Design review of the part built by this model. Coordinates are the model's own, in mm. A direction names the side the tool comes from. Give positions to 0.01 mm unless a question says otherwise; leave off trailing zeros.
```python
from build123d import *

# Parameters (mm, degrees)
SKETCH1_W                        = 112
SKETCH1_H                        = 39
BOSS_EXTRUDE1_DEPTH              = 6
CUT_EXTRUDE1_REACH               = 70.505
TAP_DRILL_FOR_M3_TAP1_AT_2_COUNT = 2
TAP_DRILL_FOR_M3_TAP1_AT_2_PITCH = 30
FILLET1_R                        = 3
FILLET1_OF_MIRROR1_R             = 3
TAP_DRILL_FOR_M2_TAP1_D          = 1.6


with BuildPart() as part:
    # Sketch1 → Boss-Extrude1 (new body)
    with BuildSketch(Plane.XY):
        with Locations((0, 19.5)):
            Rectangle(SKETCH1_W, SKETCH1_H)
    extrude(amount=BOSS_EXTRUDE1_DEPTH)

    # Sketch2 → Cut-Extrude1 (cut, up to next)
    with BuildSketch(Plane.XY.offset(6), mode=Mode.PRIVATE) as cut_extrude1_sk1:
        Polygon((-56, 33), (-43.052558883, 33), (-29.196152423, 9), (-56, 9), align=None)
    cut_extrude1_tool1 = extrude(cut_extrude1_sk1.sketch, amount=-CUT_EXTRUDE1_REACH, mode=Mode.PRIVATE) & part.part
    # Sketch2 → Cut-Extrude1 (cut, up to next)
    with BuildSketch(Plane.XY.offset(6), mode=Mode.PRIVATE) as cut_extrude1_sk2:
        Polygon((-39.588457268, 39), (-37.856406461, 36), (-19.814954576, 36), (-10, 19), (0, 19), (0, 39), align=None)
    cut_extrude1_tool2 = extrude(cut_extrude1_sk2.sketch, amount=-CUT_EXTRUDE1_REACH, mode=Mode.PRIVATE) & part.part
    # Sketch2 → Cut-Extrude1 (cut, up to next)
    with BuildSketch(Plane.XY.offset(6), mode=Mode.PRIVATE) as cut_extrude1_sk3:
        Polygon((-56, 3), (-25.732050808, 3), (-24, 0), (-56, 0), align=None)
    cut_extrude1_tool3 = extrude(cut_extrude1_sk3.sketch, amount=-CUT_EXTRUDE1_REACH, mode=Mode.PRIVATE) & part.part
    # Sketch2 → Cut-Extrude1 (cut, up to next)
    with BuildSketch(Plane.XY.offset(6), mode=Mode.PRIVATE) as cut_extrude1_sk4:
        Polygon((-13.464101615, 13), (0, 13), (0, 6), (-20.535898385, 6), (-34.392304845, 30), (-23.279056191, 30), align=None)
    cut_extrude1_tool4 = extrude(cut_extrude1_sk4.sketch, amount=-CUT_EXTRUDE1_REACH, mode=Mode.PRIVATE) & part.part
    cut_extrude1_1 = cut_extrude1_tool1.solids().sort_by_distance((-45.659675, 19.60569, 6))[0]
    add(cut_extrude1_1, mode=Mode.SUBTRACT)
    cut_extrude1_2 = cut_extrude1_tool2.solids().sort_by_distance((-11.382019, 31.286174, 6))[0]
    add(cut_extrude1_2, mode=Mode.SUBTRACT)
    cut_extrude1_3 = cut_extrude1_tool3.solids().sort_by_distance((-40.428998, 1.486092, 6))[0]
    add(cut_extrude1_3, mode=Mode.SUBTRACT)
    cut_extrude1_4 = cut_extrude1_tool4.solids().sort_by_distance((-18.182863, 16.08438, 6))[0]
    add(cut_extrude1_4, mode=Mode.SUBTRACT)
    cut_extrude1 = cut_extrude1_1 + cut_extrude1_2 + cut_extrude1_3 + cut_extrude1_4  # Cut-Extrude1 as one shape, for the pattern or mirror that repeats it

    # Sketch3 → Tap Drill for M3 Tap1 (revolve, cut)
    with BuildSketch(Plane(origin=(-56, 36, 3), x_dir=(0, 0, 1), z_dir=(0, 1, 0))):
        Polygon((0, 0), (0, 10.751075774), (1.25, 10), (1.25, 0), align=None)
    tap_drill_for_m3_tap1 = revolve(axis=Axis((-62.35, 36, 3), (1, 0, 0)), mode=Mode.SUBTRACT)

    # Tap Drill for M3 Tap1 at 2: Tap Drill for M3 Tap1 ×2
    with Locations(*[(0, -i * TAP_DRILL_FOR_M3_TAP1_AT_2_PITCH, 0) for i in range(1, TAP_DRILL_FOR_M3_TAP1_AT_2_COUNT)]):
        add(tap_drill_for_m3_tap1, mode=Mode.SUBTRACT)

    # Fillet1
    fillet1_edges = [part.edges().sort_by_distance(p)[0] for p in [
        (-43.052558883, 33, 3),
        (-29.196152423, 9, 3),
        (-39.588457268, 39, 3),
        (-10, 19, 3),
        (-19.814954576, 36, 3),
        (-37.856406461, 36, 3),
        (-23.279056191, 30, 3),
        (-13.464101615, 13, 3),
        (-20.535898385, 6, 3),
        (-34.392304845, 30, 3),
        (-25.732050808, 3, 3),
        (-24, 0, 3),
    ]]
    fillet(fillet1_edges, radius=FILLET1_R - 0.0001)  # a hair under: the kernel refuses the full size

    # Mirror1: Cut-Extrude1, Tap Drill for M3 Tap1 across plane
    add(cut_extrude1.mirror(Plane(origin=(0, 0, 0), x_dir=(0, 0, 1), z_dir=(1, 0, 0))), mode=Mode.SUBTRACT)
    add(tap_drill_for_m3_tap1.mirror(Plane(origin=(0, 0, 0), x_dir=(0, 0, 1), z_dir=(1, 0, 0))), mode=Mode.SUBTRACT)

    # Mirror1 copy 1 sketch → Mirror1 copy 1 (revolve, cut)
    with BuildSketch(Plane(origin=(56, 6, 3), x_dir=(0, 0, 1), z_dir=(0, 1, 0))):
        Polygon((0, 0), (0, -10.751075774), (1.25, -10), (1.25, 0), align=None)
    revolve(axis=Axis((62.35, 6, 3), (1, 0, 0)), mode=Mode.SUBTRACT)

    # Fillet1 of Mirror1
    fillet1_of_mirror1_edges = [part.edges().sort_by_distance(p)[0] for p in [
        (43.052558883, 33, 3),
        (29.196152423, 9, 3),
        (39.588457268, 39, 3),
        (10, 19, 3),
        (19.814954576, 36, 3),
        (37.856406461, 36, 3),
        (23.279056191, 30, 3),
        (13.464101615, 13, 3),
        (20.535898385, 6, 3),
        (34.392304845, 30, 3),
        (25.732050808, 3, 3),
        (24, 0, 3),
    ]]
    fillet(fillet1_of_mirror1_edges, radius=FILLET1_OF_MIRROR1_R - 0.0001)  # a hair under: the kernel refuses the full size

    # Tap Drill for M2 Tap1 (through all)
    with Locations(Plane.XY.offset(6)):
        with Locations((-19.6, 3), (0, 3), (19.6, 3)):
            Hole(TAP_DRILL_FOR_M2_TAP1_D / 2)


solid = part.part
```
1. Machinability: for faces 1 (the face through (-51.07, 37.109, 3.577)), 2 (the face through (20.07, 35.61, 2.96)), 3 (the face through (-42, 3, 3)), 4 (the face through (50, 33, 3)), 5 (the face through (27, 30, 3)), which of the approach directions +Z, -Z, +X, -X, +Y, -Y give a long, thin tool a straight path to every point of the face, cutting with its end or side? Answer none if there is none.
Recorded:
face 1: -X
face 2: +Z, -Z, +Y
face 3: +Z, -Z, -X, -Y
face 4: +Z, -Z, +X
face 5: +Z, -Z
2. Draft analysis for pull direction Z (two halves, no side actions). For faces 6 (the face through (51.07, 7.109, 3.577)), 7 (the face through (0, 15, 0)), 8 (the face through (0, 15, 6)), state which applies: pulls with the +Z half, pulls with the -Z half, needs draft (parallel to the pull), parting line crosses it, or undercut.
Recorded:
face 6: undercut
face 7: pulls with the -Z half
face 8: pulls with the +Z half
3. For pin 1 (1.8 mm diameter, centred on x = -49.5, z = 3, fed in from -Y); pin 2 (3.5 mm diameter, centred on x = 26.5, z = 3, fed in from -Y); pin 3 (2.5 mm diameter, centred on x = -19.6, y = 3, fed in from +Z); pin 4 (2 mm diameter, centred on x = 27, z = 2.5, fed in from -Y), all flat-tipped, find the tip position at first contact; note any pin that passes through.
Recorded:
pin 1: stops at y = 3
pin 2: stops at y = 1.31
pin 3: stops at z = 6
pin 4: stops at y = 2.62
4. For line 1 along Y through (x, z) = (52.75, 3); line 2 along Y through (x, z) = (0, 2.8); line 3 along Z through (x, y) = (-54, 36), list the stretches that pass through material, from the lowest coordinate up.
Recorded:
line 1: y = 3 to 4.75, 7.25 to 9, 33 to 34.75, 37.25 to 39
line 2: y = 0 to 2.2, 3.8 to 6, 13 to 19
line 3: z = 0 to 1.75, 4.25 to 6
